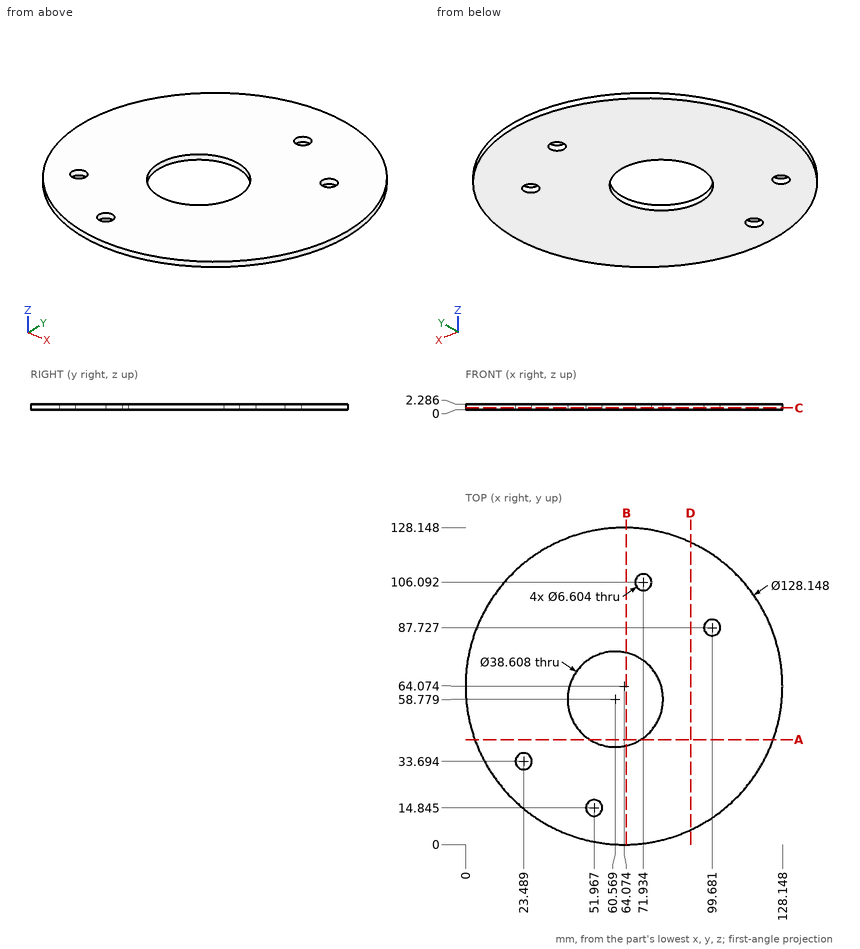
Can you work these out from the drawing? Everything is in mm from the part's minimum corner. Coordinates: 2 decimals unless noted, no trailing zeros. Write each loop counter-clockwise with the first axis right and the second up, starting at its lowest first coordinate (ties: lowest second). Pieces come first, ordered by that corner, then holes. Notation, with made-up numbers: (77, -20.75) -> (84, -20.75) arc R12 cw to (84, -7.75) -> close; hole circle Ø2 at (75, 62). An arc over 180 degrees is marked (long way). Write each question's results on one line, items separated by ' | '. Start each with the question number.
Q1. Imagine slicing it at D-D (x = 91). Write out the boundary of the cut face in (y, z) (1 decimal), then the cut area to 3 significant figures.
Q2. Imagine slicing it at C-C (z = 0.7). Write out the boundary of the cut face in (x, y) (1 decimal).
Q3. If I drill on probe 1 along Y at (x, z) = (70.5, 1.35) (1 decimal); probe 2 along Y at (x, z) = (51, 0.2) (1 decimal); probe 3 along Y at (x, z) = (25, 1) (1 decimal), over which ranges is the centre line in solid material (lowest first)?
Q4. Imagine slicing it at A-A (y = 42.5). Write out the boundary of the cut face in (x, z) (1 decimal).
Q5. Imagine slicing it at B-B (x = 65). Write out the boundary of the cut face in (y, z).
Q6. I'm going to push a flat-ended pin straight in: pin 1 (8.5 mm diameter, centred on x = 23.49, y = 33.69, fed in from -Z). Where does the tip first touch, or does it pass through?
Taken from the geometry:
1) outline: (5.9, 0) -> (122.2, 0) -> (122.2, 2.3) -> (5.9, 2.3) -> close | area: 266 mm^2
2) outline: circle Ø128.1 at (64.1, 64.1); hole circle Ø6.6 at (23.5, 33.7); hole circle Ø38.6 at (60.6, 58.8); hole circle Ø6.6 at (52, 14.8); hole circle Ø6.6 at (71.9, 106.1); hole circle Ø6.6 at (99.7, 87.7)
3) probe 1: y = 0.3 to 42.2, 75.3 to 103.1, 109.1 to 127.8 | probe 2: y = 1.3 to 11.7, 18 to 42, 75.5 to 126.8 | probe 3: y = 13.3 to 30.8, 36.6 to 114.9
4) outline: (3.7, 0) -> (50.2, 0) -> (50.2, 2.3) -> (3.7, 2.3) -> close; (70.9, 0) -> (124.4, 0) -> (124.4, 2.3) -> (70.9, 2.3) -> close
5) outline: (0.01, 0) -> (39.99, 0) -> (39.99, 2.29) -> (0.01, 2.29) -> close; (77.57, 0) -> (128.14, 0) -> (128.14, 2.29) -> (77.57, 2.29) -> close
6) pin 1: stops at z = 0
